For this review, take the finished solid that the model builds, in its own axes (mm). Give positions to 0.01 mm unless a question says otherwise; leave off trailing zeros. Write each loop counter-clockwise with the first axis right and the second up, starting at its lowest first coordinate (ties: lowest second). Pieces come first, ordered by that corner, then holes. Notation, with made-up numbers: (53, 52) -> (86, 52) arc R23 cw to (86, 87) -> close; hole circle Ø1 at (88, 12). An arc over 180 degrees is marked (long way). Write item = value, one per line.
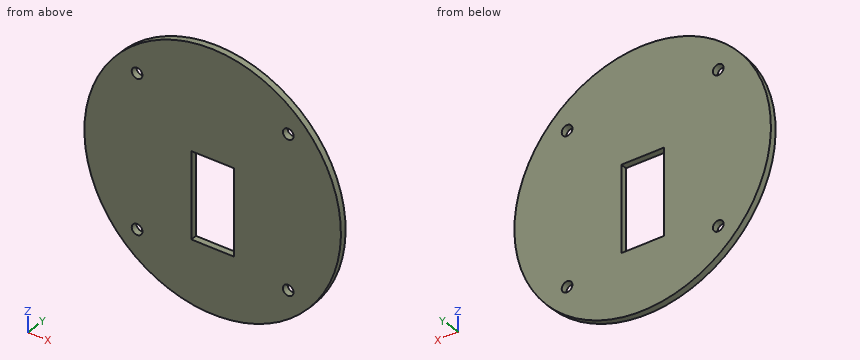
```python
from build123d import *

# Parameters (mm, degrees)
SKETCH_1_R      = 60
SKETCH_1_R_2    = 2.5
SKETCH_1_W      = 20
SKETCH_1_H      = 40
EXTRUDE_1_DEPTH = 3


with BuildPart() as part:
    # 草图1 → 凸台-拉伸1 (new body)
    with BuildSketch(Plane(origin=(0, 0, 0), x_dir=(1, 0, 0), z_dir=(0, 1, 0))):
        with Locations(Location((0, 0, 0), (0, 0, 270))):
            Circle(SKETCH_1_R)
        with Locations(Location((-35.355339059, 35.355339059, 0), (0, 0, 270))):
            Circle(SKETCH_1_R_2, mode=Mode.SUBTRACT)
        with Locations(Location((35.355339059, 35.355339059, 0), (0, 0, 270))):
            Circle(SKETCH_1_R_2, mode=Mode.SUBTRACT)
        with Locations(Location((35.355339059, -35.355339059, 0), (0, 0, 270))):
            Circle(SKETCH_1_R_2, mode=Mode.SUBTRACT)
        with Locations(Location((-35.355339059, -35.355339059, 0), (0, 0, 270))):
            Circle(SKETCH_1_R_2, mode=Mode.SUBTRACT)
        with Locations((0, 10)):
            Rectangle(SKETCH_1_W, SKETCH_1_H, mode=Mode.SUBTRACT)
    extrude(amount=EXTRUDE_1_DEPTH)


solid = part.part
```
(1) Take a section at C-C (y = 1.05). Write out the cut boundary in (x, z).
Answers below:
outline = circle Ø120 at (0, 0); hole circle Ø5 at (-35.36, -35.36); hole circle Ø5 at (-35.36, 35.36); hole (-10, -30) -> (10, -30) -> (10, 10) -> (-10, 10) -> close; hole circle Ø5 at (35.36, -35.36); hole circle Ø5 at (35.36, 35.36)
(2) Take a section at D-D (x = 39.5). Write out the cut boundary in (y, z), plus the area to 3 significant figures.
Answers below:
outline = (0, -45.16) -> (3, -45.16) -> (3, 45.16) -> (0, 45.16) -> close
area = 271 mm^2
(3) Take a section at B-B (z = 0). Write out the cut boundary in (x, y).
Answers below:
outline = (-60, 0) -> (-10, 0) -> (-10, 3) -> (-60, 3) -> close; (10, 0) -> (60, 0) -> (60, 3) -> (10, 3) -> close
(4) To check wall thickness, follow probe 1 along X at (y, z) = (0.5, 35); probe 2 along Z at (x, y) = (1, 2.05); probe 3 along X at (y, z) = (0.3, -36). State the ranges of each line that lie inside material, in increasing order.
Answers below:
probe_1 = -48.73 to -37.83, -32.88 to 32.88, 37.83 to 48.73
probe_2 = -59.99 to -30, 10 to 59.99
probe_3 = -48 to -37.77, -32.94 to 32.94, 37.77 to 48
(5) For pin 1 (1.5 mm diameter, centred on y = 1, z = -4, fed in from -X); pin 2 (1.5 mm diameter, centred on x = 2, y = 1.5, fed in from -Z), all flat-tipped, find the tip position at first contact; note any pin that passes through.
Answers below:
pin_1 = -59.91
pin_2 = -59.99
(6) Take a section at A-A (x = 0). Write out the cut boundary in (y, z), plus the area to 3 significant figures.
Answers below:
outline = (0, -60) -> (3, -60) -> (3, -30) -> (0, -30) -> close; (0, 10) -> (3, 10) -> (3, 60) -> (0, 60) -> close
area = 240 mm^2
